Design review of the part shown in the three views and the two pictorial views. Dimensions are in mm from the part's minimum x, y and z. Coordinates: 2 decimals unless noted, no trailing zeros. Write each loop counter-clockwise with the first axis right and the second up, starting at its lowest first coordinate (ties: lowest second). Pieces come first, ordered by that corner, then holes.
Q1. For L1, parallel to Z at x = 0.55, y = 2.15 (1 decimal); L2, parallel to Y at x = 1.55, z = 7.5; L3, parallel to X at y = 0.45, z = 4.75 (1 decimal), list the stretches that pass through material, from the lowest coordinate up.
Q2. Take a section at B-B, the plane z = 4. Write out the cut boundary in (x, y).
Q3. Take a section at A-A, the plane y = 0.4. State how many separate pieces and enclosed holes the cut face has.
Q4. The part is to be moulded in two halves that separate along X. For the marked faces 1 and 2, say which applies: released by +X, released by -X, zero draft, split by the parting line, or undercut.
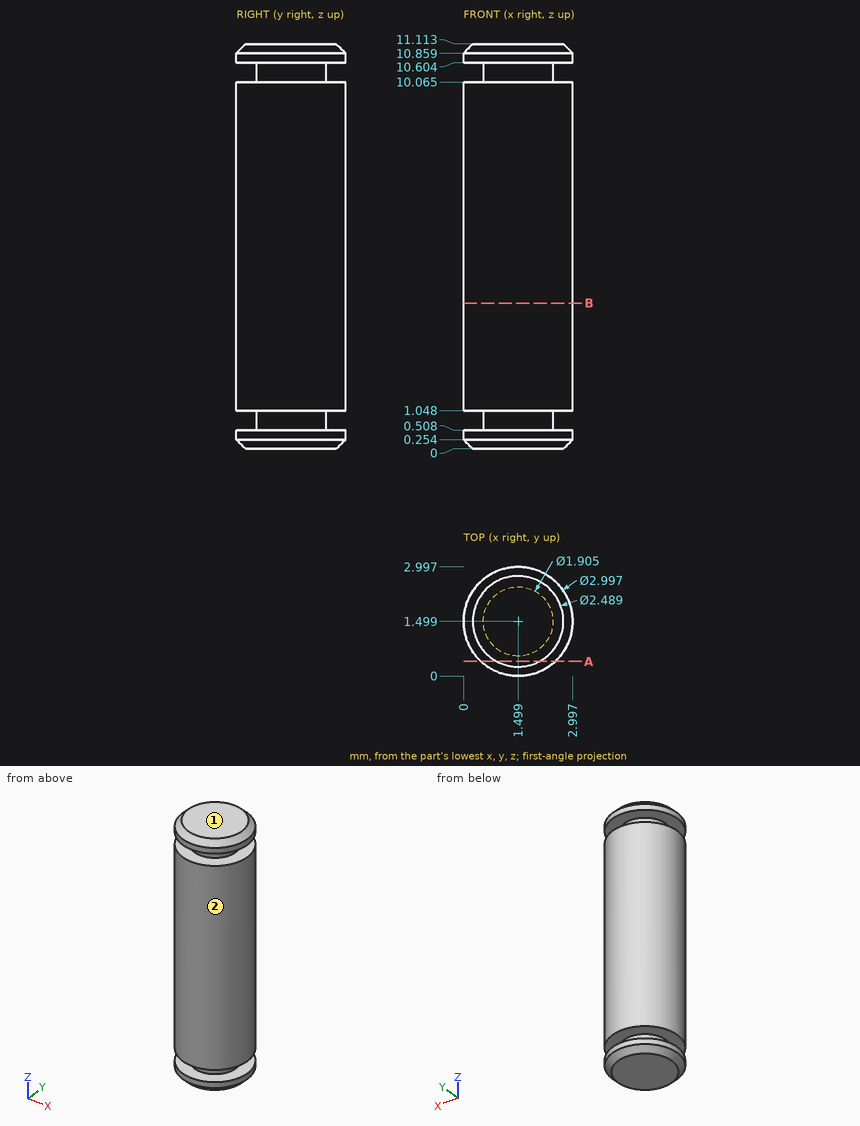
Responses:
1. L1: z = 0 to 0.5, 1 to 10.1, 10.6 to 11.1
1. L2: y = 0 to 3
1. L3: x = 0.4 to 2.6
2. outline: circle Ø3 at (1.5, 1.5)
3. separate pieces: 3
3. enclosed holes: 0
4. face 1: zero draft
4. face 2: split by the parting line
